Verification items for this drawing (mm, ordinates from the low corner). A direction names the side the tool comes from. Round coordinates to 2 decimals unless told otherwise and drop trailing zeros. Loops run counter-clockwise (first coordinate to the right, second up) from the corner with the lowest first, then second, coordinate; pieces in that order, holes last. Notation, with made-up numbers: M -25,47.5 L -7,47.5 A36 cw -7,85.5 Z; hole C 53.5,-23 d1. An arc over 180 degrees is marked long. Write item = value, one per line. Start each with the question number.
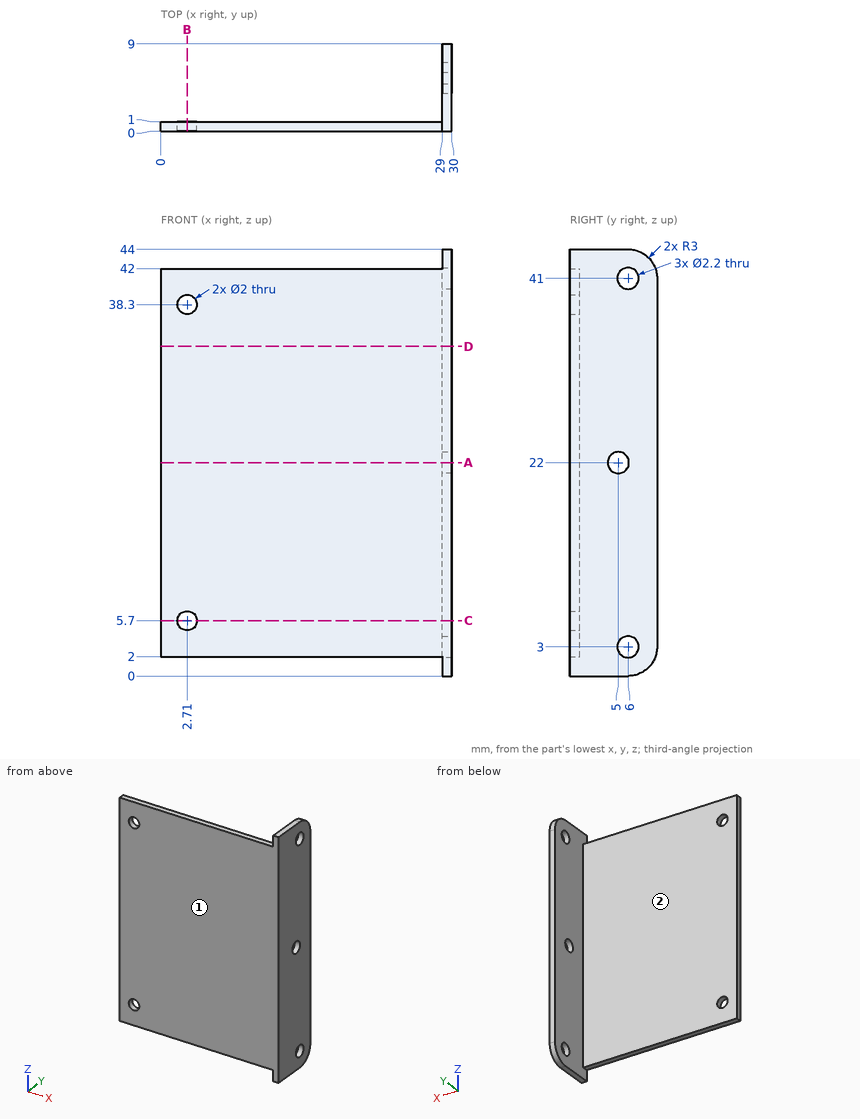
1. Section check C-C, the plane z = 5.7. Enter the section's corners in (x, y).
2. Section check B-B, the plane x = 2.71. Enter the section's corners in (y, z).
3. Section check A-A, the plane z = 22. Enter the section's corners in (x, y).
4. Gauge pin test, flat ends, axial feed: P1, Ø3, axis at y = 6, z = 41, coming from the -X side; P2, Ø2.5, axis at x = 2.71, z = 38.3, coming from the +Y side; P3, Ø2.5, axis at y = 6, z = 3, coming from the +X side. Record the tip position at first contact, or that the pin passes through.
5. Thickness scan on line 1 (Z direction, x = 2.71, y = 0.5); line 2 (Y direction, x = 29.4, z = 22); line 3 (X direction, y = 0.35, z = 38.3). Record the ranges inside material, lowest first.
6. Tool access check on the marked faces 1 and 2. Record the directions out of +Z, -Z, +X, -X, +Y, -Y that give a thin tool (end or side, any length) a straight path to the whole face; none if there is none.
7. Section check D-D, the plane z = 34. Enter the section's corners in (x, y), and give its area (3 significant figures).
Computed values:
q1.outline = M 0,0 L 1.71,0 L 1.71,1 L 0,1 Z; M 3.71,0 L 30,0 L 30,9 L 29,9 L 29,1 L 3.71,1 Z
q2.outline = M 0,2 L 1,2 L 1,4.7 L 0,4.7 Z; M 0,6.7 L 1,6.7 L 1,37.3 L 0,37.3 Z; M 0,39.3 L 1,39.3 L 1,42 L 0,42 Z
q3.outline = M 0,0 L 30,0 L 30,3.9 L 29,3.9 L 29,1 L 0,1 Z; M 29,6.1 L 30,6.1 L 30,9 L 29,9 Z
q4.P1 = 29
q4.P2 = 1
q4.P3 = 30
q5.line_1 = 2 to 4.7, 6.7 to 37.3, 39.3 to 42
q5.line_2 = 0 to 3.9, 6.1 to 9
q5.line_3 = 0 to 1.71, 3.71 to 30
q6.face_1 = +Z, -Z, +X, -X, -Y
q6.face_2 = +Z, -Z, -X, +Y
q7.outline = M 0,0 L 30,0 L 30,9 L 29,9 L 29,1 L 0,1 Z
q7.area = 38.0 mm2
